Source: CAD feature listing. Evaluate the final solid. Frame: model axes, mm. Face numbers are marked on the shaded views. Coordinates: 2 decimals unless noted, no trailing zeros. Loops run counter-clockwise (first coordinate to the right, second up) from the corner with the lowest first, then second, coordinate; pieces in that order, holes last. Notation, with made-up numbers: M 6.25,-15.5 L 26.25,-15.5 A34 ccw 26.25,23.5 Z; hole C -37.75,34 d7. An arc over 180 degrees is marked long. One line per question, with ' | ' between items. Start each with the question number.
1. Section query C-C, the plane y = -9.75. Output: boundary loops of the cut face in (x, z).
2. Section query D-D, the plane z = 5.5. Output: boundary loops of the cut face in (x, y).
3. Section query A-A, the plane z = 0. Output: boundary loops of the cut face in (x, y), and give its area (4 significant figures).
4. Mould query, pull axis Z, two halves, no side actions, for the marked faces 1 and 2. Classes: pulls with the +Z half, pulls with the -Z half, needs draft (parallel to the pull), parting line crosses it, or undercut.
5. Ray query, probe 1 along Z at (x, y) = (0, 4); probe 2 along X at (y, z) = (-8.25, 0); probe 3 along Y at (x, z) = (6.5, -0.25). Return the intervals inside material, ascending.
6. Pin query (flat end, axial travel): P1, Ø1.5, axis at y = -10, z = -2.5, coming from the -X side; P2, Ø7.5, axis at x = -2, z = -2, coming from the -Y side; P3, Ø6, axis at y = 0.5, z = 4.5, coming from the +X side. Return the tip coordinate at first contact, or that it passes through.
7. Section query B-B, the plane x = 0. Output: boundary loops of the cut face in (y, z).
```python
from build123d import *

# Parameters (mm, degrees)
F0_R     = 15
F0_R_2   = 7.55
F1_DEPTH = 15
F2_R     = 15
F2_R_2   = 2.5
F3_DEPTH = 5
F5_DEPTH = 15


with BuildPart() as f1:
    # F0 (on Front) → F1 (new body)
    with BuildSketch(Plane.XZ):
        Circle(F0_R)
        Circle(F0_R_2, mode=Mode.SUBTRACT)
    extrude(amount=F1_DEPTH)

    # F2 (on face) → F3 (join)
    with BuildSketch(Plane(origin=(0, 0, 0), x_dir=(-1, 0, 0), z_dir=(0, 1, 0))):
        Circle(F2_R)
        Circle(F2_R_2, mode=Mode.SUBTRACT)
    extrude(amount=F3_DEPTH)

    # F4 (on face) → F5 (join)
    with BuildSketch(Plane.XZ.offset(15)):
        with BuildLine():
            ThreePointArc((7.399493, -1.5), (7.55, 0), (7.399493, 1.5))
            Line((7.399493, 1.5), (6.55, 1.5))
            Line((6.55, 1.5), (6.55, -1.5))
            Line((6.55, -1.5), (7.399493, -1.5))
        make_face()
    extrude(amount=-F5_DEPTH)


solid = f1.part
```
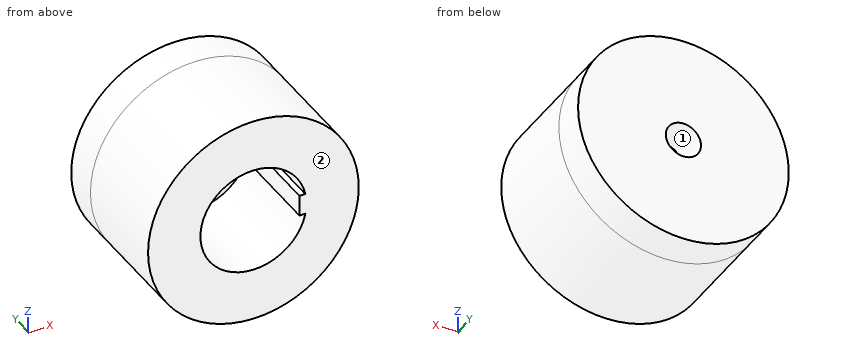
Taken from the geometry:
1) outline: C 0,0 d30; hole M 6.55,-1.5 L 6.55,1.5 L 7.4,1.5 A7.55 ccw long 7.4,-1.5 Z
2) outline: M -13.96,-15 L -5.17,-15 L -5.17,0 L 5.17,0 L 5.17,-15 L 13.96,-15 L 13.96,5 L -13.96,5 Z
3) outline: M -15,-15 L -7.55,-15 L -7.55,0 L -2.5,0 L -2.5,5 L -15,5 Z; M 2.5,0 L 6.55,0 L 6.55,-15 L 15,-15 L 15,5 L 2.5,5 Z | area: 363.5 mm^2
4) face 1: undercut | face 2: needs draft
5) probe 1: -15 to -2.5, 2.5 to 15 | probe 2: -15 to -7.55, 6.55 to 15 | probe 3: 0 to 5
6) P1: x = -14.9 | P2: y = 0 | P3: x = 14.92
7) outline: M -15,-15 L 5,-15 L 5,-2.5 L 0,-2.5 L 0,-7.55 L -15,-7.55 Z; M -15,7.55 L 0,7.55 L 0,2.5 L 5,2.5 L 5,15 L -15,15 Z
